Could you check a few things on this model? Use its own coordinates, in mm. Coordinates: 2 decimals unless noted, no trailing zeros. Loops run counter-clockwise (first coordinate to the right, second up) from the corner with the lowest first, then second, coordinate; pieces in that order, holes last. Notation, with made-up numbers: (77, 73) -> (132, 73) arc R28 ccw to (132, 93) -> close; hole circle Ø3 at (43, -6.75). An arc over 180 degrees is marked (long way). One line per question, with ' | ' between items. Start each with the question number.
(1) If we mould it in two halves opening along X, with no side actions, what happens to faces 1 (the face through (-0.867, -3.905, -0.493)), 2 (the face through (4, 2, 0))? For each: pulls with the +X half, pulls with the -X half, needs draft (parallel to the pull), parting line crosses it, or undercut.
(2) I'm going to push flat-ended pins straight in: pin 1 Ø8 at (y, z) = (-7, 17) entering from +X; pin 2 Ø5 at (x, z) = (-3, 30) entering from -Y; pin 3 Ø5 at (y, z) = (-3, 38.5) entering from +X. Where does each tip first touch, or does it pass through?
(3) Suppose I cut it at A-A (z = 53). Please give me the cut outline in (x, y), plus the area to 3 significant figures.
(4) If I drill on line 1 along Z through (x, y) = (-8, 2); line 2 along X through (y, z) = (0.5, 18); line 3 along X through (y, z) = (4, 52), over which ranges is the centre line in solid material (lowest first)?
Autodesk Inventor part; units mm, degrees
ref_plane "YZ Plane" through (0, 0, 0) normal (1, 0, 0) x (0, 1, 0)
ref_plane "XZ Plane" through (0, 0, 0) normal (0, 1, 0) x (-1, 0, 0)
ref_plane "XY Plane" through (0, 0, 0) normal (0, 0, 1) x (1, 0, 0)
sketch "Skizze1" plane through (0, 0, 0) normal (0, 0, 1) x (1, 0, 0)
  circle A0 centre (0, 0) radius 9.15
  circle A1 centre (0, 0) radius 4
  dimension "d0" = 18.3
  dimension "d3" = 8
extrude "Extrusion1" add sketch "Skizze1" along normal blind 65.1 contours A0 | A1
extrude "Extrusion2" add sketch "Skizze1" against normal blind 1 contours A1
fillet "Rundung1" radius 1 2 edges at (-9.15, 0, 0) (-9.15, 0, 65.1)
properties part number "LG INR18650MJ1" material "Kupfer, Guss"
Checks:
1) face 1: parting line crosses it | face 2: needs draft
2) pin 1: stops at x = 8.64 | pin 2: stops at y = -9.14 | pin 3: stops at x = 9.14
3) outline: circle Ø18.3 at (0, 0) | area: 263 mm^2
4) line 1: z = 0 to 65.1 | line 2: x = -9.14 to 9.14 | line 3: x = -8.23 to 8.23
